from build123d import *

# Parameters (mm, degrees)
F0_W     = 102.5
F0_H     = 51
F1_DEPTH = 25
F2_W     = 90
F2_H     = 40
F3_DEPTH = 12.5


# Not quite as in the source:
# - the program builds the solid bodies; features that only make, move or delete a surface that nothing else refers to are left out


with BuildPart() as f1:
    # F0 (on Front) → F1 (new body)
    with BuildSketch(Plane.XZ):
        Rectangle(F0_W, F0_H)
    extrude(amount=F1_DEPTH)

    # F2 (on face) → F3 (cut, symmetric)
    with BuildSketch(Plane.XZ.offset(25)):
        Rectangle(F2_W, F2_H)
    extrude(amount=F3_DEPTH, both=True, mode=Mode.SUBTRACT)


solid = f1.part
Here's how the part is built. I have some questions about the finished solid (model axes, mm). A direction names the side the tool comes from. Coordinates: 2 decimals unless noted, no trailing zeros. Order: outer loops, then holes, each group sorted by start corner. A loop starts at its lowest first (then second) coordinate and runs counter-clockwise, first axis right, second up.
Item 1: For P1, Ø4, axis at x = -28.5, z = -9, coming from the -Y side; P2, Ø5, axis at x = 19.5, z = -11, coming from the +Y side, each with a flat end and sliding along its axis, tell me the tip position at first contact or that it passes through.
Result sheet:
P1: stops at y = -12.5
P2: stops at y = 0
Item 2: If we section it at A-A on x = -22: List the corners of the cut face in (y, z) for me, plus the area to 3 significant figures.
Result sheet:
outline: (-25, -25.5) - (0, -25.5) - (0, 25.5) - (-25, 25.5) - (-25, 20) - (-12.5, 20) - (-12.5, -20) - (-25, -20) - close
area: 775 mm2
Item 3: For faces 4 (the face through (-1, -12, 25.5)), 5 (the face through (-1, -12.5, 0)), which set-ups out of +Z, -Z, +X, -X, +Y, -Y let a thin tool reach every point of the face, with its end or its side?
Result sheet:
face 4: +Z, +X, -X, +Y, -Y
face 5: -Y
Item 4: If we section it at C-C on y = -21.25: List the corners of the cut face in (x, z) for me.
Result sheet:
outline: (-51.25, -25.5) - (51.25, -25.5) - (51.25, 25.5) - (-51.25, 25.5) - close; hole (-45, -20) - (45, -20) - (45, 20) - (-45, 20) - close
Item 5: I need wall thicknesses on line 1 (Z direction, x = 25.5, y = -19.25); line 2 (X direction, y = -15.25, z = 9.5); line 3 (Y direction, x = 15, z = -11.5). Which ranges of each line are inside material? Lowest first, please.
Result sheet:
line 1: z = -25.5 to -20, 20 to 25.5
line 2: x = -51.25 to -45, 45 to 51.25
line 3: y = -12.5 to 0
Item 6: If we mould it in two halves opening along X, with no side actions, what happens to faces 1 (the face through (-1, -19, 20)), 2 (the face through (-1, -12, -25.5)), 3 (the face through (51.25, -12, 0))? For each: +X half, -X half, draft (parallel to the pull), parting line (faces both ways), or undercut.
Result sheet:
face 1: undercut
face 2: draft
face 3: +X half
Item 7: If we section it at B-B on z = 17.5: List the corners of the cut face in (x, y) for me, plus the area to 3 significant figures.
Result sheet:
outline: (-51.25, -25) - (-45, -25) - (-45, -12.5) - (45, -12.5) - (45, -25) - (51.25, -25) - (51.25, 0) - (-51.25, 0) - close
area: 1,440 mm2
